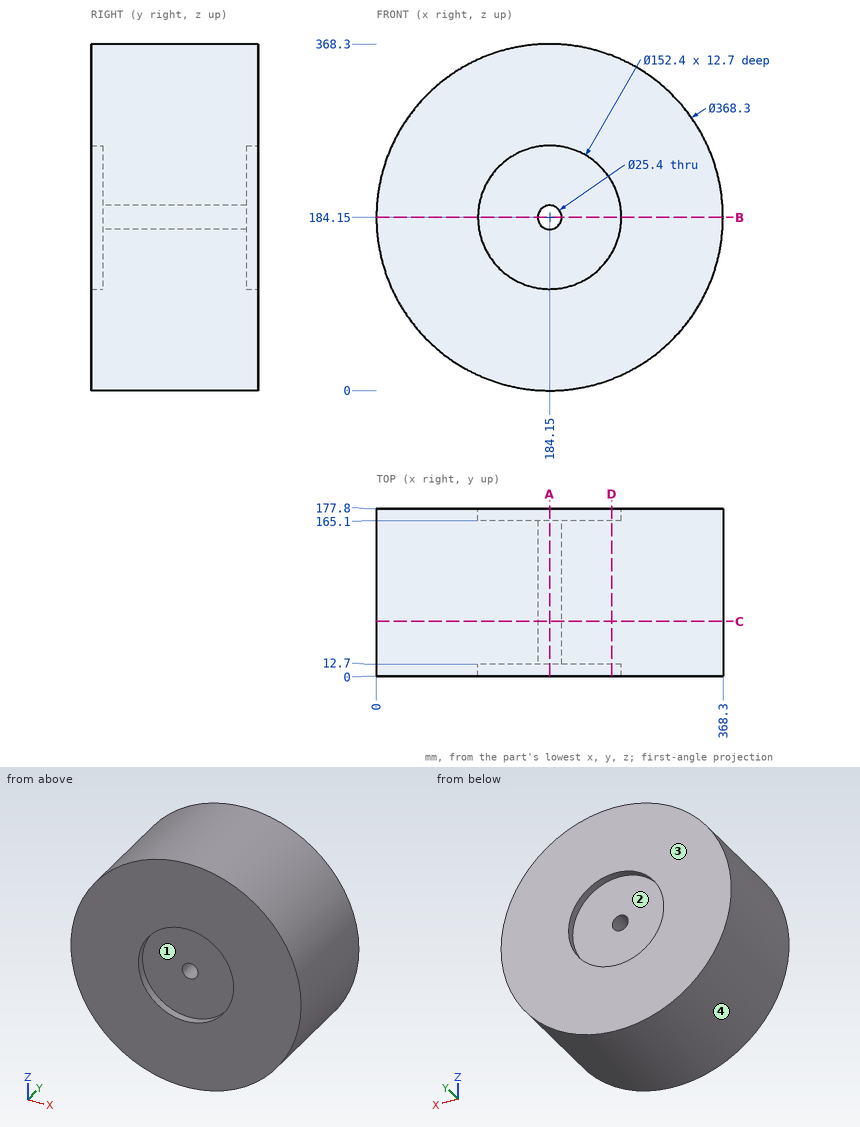
Verification items for this drawing (mm, ordinates from the low corner). Give positions to 0.01 mm unless a question says otherwise; leave off trailing zeros. Order: outer loops, then holes, each group sorted by start corner. A loop starts at its lowest first (then second) coordinate and runs counter-clockwise, first axis right, second up.
1) Draft check along X on the marked faces 1, 2, 3 and 4. Enter one of: released by +X, released by -X, zero draft, split by the parting line, or undercut.
Results are:
face 1: undercut
face 2: undercut
face 3: zero draft
face 4: split by the parting line
2) Cross-section at A-A (x = 184.15). Record the boundary of the cut face in (y, z).
Results are:
outline: (0, 0) - (177.8, 0) - (177.8, 107.95) - (165.1, 107.95) - (165.1, 171.45) - (12.7, 171.45) - (12.7, 107.95) - (0, 107.95) - close; (0, 260.35) - (12.7, 260.35) - (12.7, 196.85) - (165.1, 196.85) - (165.1, 260.35) - (177.8, 260.35) - (177.8, 368.3) - (0, 368.3) - close
3) Cross-section at C-C (y = 58). Record the boundary of the cut face in (x, z), then the cut area to 3 significant figures.
Results are:
outline: circle Ø368.3 at (184.15, 184.15); hole circle Ø25.4 at (184.15, 184.15)
area: 106,000 mm2
4) Cross-section at D-D (x = 250). Record the boundary of the cut face in (y, z), then the cut area to 3 significant figures.
Results are:
outline: (0, 12.18) - (177.8, 12.18) - (177.8, 145.81) - (165.1, 145.81) - (165.1, 222.49) - (177.8, 222.49) - (177.8, 356.12) - (0, 356.12) - (0, 222.49) - (12.7, 222.49) - (12.7, 145.81) - (0, 145.81) - close
area: 59,200 mm2
5) Gauge pin test, flat ends, axial feed: pin 1 (12 mm diameter, centred on x = 156, y = 26.5, fed in from -Z); pin 2 (1.5 mm diameter, centred on y = 49, z = 160.5, fed in from -X); pin 3 (1.5 mm diameter, centred on y = 112.5, z = 94, fed in from +X). Record the tip position at first contact, or that the pin passes through.
Results are:
pin 1: stops at z = 1.34
pin 2: stops at x = 1.43
pin 3: stops at x = 345.14
6) Material ranges on probe 1 along Z at (x, y) = (184, 5); probe 2 along Z at (x, y) = (184, 68); probe 3 along Y at (x, z) = (209, 170.5), recorded low to high.
Results are:
probe 1: z = 0 to 107.95, 260.35 to 368.3
probe 2: z = 0 to 171.45, 196.85 to 368.3
probe 3: y = 12.7 to 165.1
7) Cross-section at B-B (z = 184.15). Record the boundary of the cut face in (x, y), then the cut area to 3 significant figures.
Results are:
outline: (0, 0) - (107.95, 0) - (107.95, 12.7) - (171.45, 12.7) - (171.45, 165.1) - (107.95, 165.1) - (107.95, 177.8) - (0, 177.8) - close; (196.85, 12.7) - (260.35, 12.7) - (260.35, 0) - (368.3, 0) - (368.3, 177.8) - (260.35, 177.8) - (260.35, 165.1) - (196.85, 165.1) - close
area: 57,700 mm2
